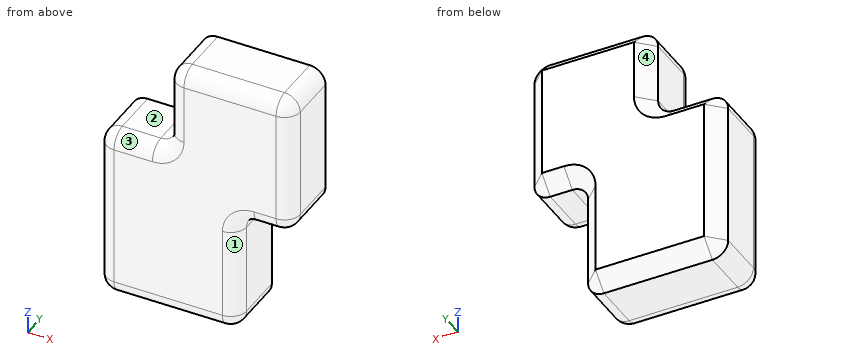
from build123d import *

# Parameters (mm, degrees)
F1_DEPTH = 25
F2_R     = 5
F3_SIZE  = 4.99999


# Not quite as in the source:
# - a fillet or chamfer is up to 0.001 mm smaller than in the source, because OpenCascade refuses the exact size


with BuildPart() as f1:
    # F0 (on Front) → F1 (new body)
    with BuildSketch(Plane.XZ):
        with BuildLine():
            Line((-4.1428460926, 16.4471715689), (-16.3246531785, 16.4471715689))
            ThreePointArc((-16.3246531785, 16.4471715689), (-19.8601870844, 14.9827054748), (-21.3246531785, 11.4471715689))
            Line((-21.3246531785, 11.4471715689), (-21.3246531785, -33.7977808714))
            ThreePointArc((-21.3246531785, -33.7977808714), (-19.8601870844, -37.3333147773), (-16.3246531785, -38.7977808714))
            Line((-16.3246531785, -38.7977808714), (18.0389609933, -38.7977808714))
            ThreePointArc((18.0389609933, -38.7977808714), (21.5744948992, -37.3333147773), (23.0389609933, -33.7977808714))
            Line((23.0389609933, -33.7977808714), (23.0389609933, -5))
            ThreePointArc((23.0389609933, -5), (24.5034270874, -1.4644660941), (28.0389609933, 0))
            Line((28.0389609933, 0), (35.034160018, 0))
            ThreePointArc((35.034160018, 0), (38.5696939239, 1.4644660941), (40.034160018, 5))
            Line((40.034160018, 5), (40.034160018, 40.125707984))
            ThreePointArc((40.034160018, 40.125707984), (38.5696939239, 43.6612418899), (35.034160018, 45.125707984))
            Line((35.034160018, 45.125707984), (5.8571539074, 45.125707984))
            ThreePointArc((5.8571539074, 45.125707984), (2.3216200015, 43.6612418899), (0.8571539074, 40.125707984))
            Line((0.8571539074, 40.125707984), (0.8571539074, 21.4471715689))
            ThreePointArc((0.8571539074, 21.4471715689), (-0.6073121866, 17.9116376629), (-4.1428460926, 16.4471715689))
        make_face()
    extrude(amount=F1_DEPTH)

    # F2
    f2_edges = [f1.edges().sort_by_distance(p)[0] for p in [
        (0.857154, -25, -38.797781),
    ]]
    fillet(f2_edges, radius=F2_R)

    # F3 (size 5 in the source; OpenCascade refuses exactly that, so slightly less here)
    f3_edges = [f1.edges().sort_by_distance(p)[0] for p in [
        (20.445657, 0, 45.125708),
        (2.32162, 0, 43.661242),
        (0.857154, 0, 30.78644),
        (-0.607312, 0, 17.911638),
        (-10.23375, 0, 16.447172),
        (-19.860187, 0, 14.982705),
        (-21.324653, 0, -11.175305),
        (-19.860187, 0, -37.333315),
        (0.857154, 0, -38.797781),
        (21.574495, 0, -37.333315),
        (23.038961, 0, -19.39889),
        (24.503427, 0, -1.464466),
        (31.536561, 0, 0),
        (38.569694, 0, 1.464466),
        (40.03416, 0, 22.562854),
        (38.569694, 0, 43.661242),
    ]]
    chamfer(f3_edges, length=F3_SIZE)


solid = f1.part
Verification items for the finished model (mm, model axes). Face numbers are marked on the shaded views. A direction names the side the tool comes from. Coordinates: 2 decimals unless noted, no trailing zeros. Order: outer loops, then holes, each group sorted by start corner. A loop starts at its lowest first (then second) coordinate and runs counter-clockwise, first axis right, second up. Notation, with made-up numbers: M 77,-1.75 L 99,-1.75 A34 cw 99,31.25 Z; hole C 7.5,38.25 d11. An arc over 180 degrees is marked long. One line per item, written item: value. Start each with the question number.
Item 1: Sectioned sample at A-A (y = -8.75). Enter the section's corners in (x, z).
Item 2: Sectioned sample at C-C (x = 9.5). Enter the section's corners in (y, z).
Item 3: Scan lines: probe 1 along X at (y, z) = (-12.5, -24); probe 2 along Z at (x, y) = (-15, -7.5); probe 3 along Z at (x, y) = (29.5, -8.75). Record each from-to range of solid material in increasing order.
Item 4: Sectioned sample at B-B (z = 26.5). Enter the section's corners in (x, y), then the cut area to 3 significant figures.
Item 5: Access from +Z, -Z, +X, -X, +Y, -Y to the whole of each face (thin tool, end or side, straight path). Record for the marked faces 1, 2, 3 and 4.
Item 6: Gauge pin test, flat ends, axial feed: pin 1 (7.5 mm diameter, centred on x = 31.5, y = -15, fed in from -Z); pin 2 (1 mm diameter, centred on y = -3.5, z = -29, fed in from +X); pin 3 (4.5 mm diameter, centred on y = -12, z = -16, fed in from +X). Record the tip position at first contact, or that the pin passes through.
Item 7: Sectioned sample at D-D (y = -3.5). Enter the section's corners in (x, z), then the cut area to 3 significant figures.
Conclusion:
1. outline: M -21.32,-33.8 A5 ccw -16.32,-38.8 L 18.04,-38.8 A5 ccw 23.04,-33.8 L 23.04,-5 A5 cw 28.04,0 L 35.03,0 A5 ccw 40.03,5 L 40.03,40.13 A5 ccw 35.03,45.13 L 5.86,45.13 A5 ccw 0.86,40.13 L 0.86,21.45 A5 cw -4.14,16.45 L -16.32,16.45 A5 ccw -21.32,11.45 Z
2. outline: M -25,-33.8 A5 ccw -20,-38.8 L -5,-38.8 L 0,-33.8 L 0,40.13 L -5,45.13 L -20,45.13 A5 ccw -25,40.13 Z
3. probe 1: x = -21.32 to 23.04
3. probe 2: z = -38.8 to 16.45
3. probe 3: z = 0 to 45.13
4. outline: M 0.86,-20 A5 ccw 5.86,-25 L 35.03,-25 A5 ccw 40.03,-20 L 40.03,-5 L 35.03,0 L 5.86,0 L 0.86,-5 Z
4. area: 944 mm^2
5. face 1: -Z, +X, -Y
5. face 2: +Z, -X, +Y, -Y
5. face 3: +Z, -X, -Y
5. face 4: +Z, -X, +Y
6. pin 1: stops at z = -0.01
6. pin 2: stops at x = 22.04
6. pin 3: stops at x = 23.04
7. outline: M -19.82,-33.8 A3.5 ccw -16.32,-37.3 L 18.04,-37.3 A3.5 ccw 21.54,-33.8 L 21.54,-5 A6.5 cw 28.04,1.5 L 35.03,1.5 A3.5 ccw 38.53,5 L 38.53,40.13 A3.5 ccw 35.03,43.63 L 5.86,43.63 A3.5 ccw 2.36,40.13 L 2.36,21.45 A6.5 cw -4.14,14.95 L -16.32,14.95 A3.5 ccw -19.82,11.45 Z
7. area: 3,430 mm^2
